Verification items for the finished model (mm, model axes). Coordinates: 2 decimals unless noted, no trailing zeros. Write each loop counter-clockwise with the first axis right and the second up, starting at its lowest first coordinate (ties: lowest second). Pieces come first, ordered by that corner, then holes. Notation, with made-up numbers: M 31.25,5 L 45.25,5 A26 cw 45.25,44 Z; hole C 71,20 d2. An arc over 180 degrees is marked long. One line per item, written item: value.
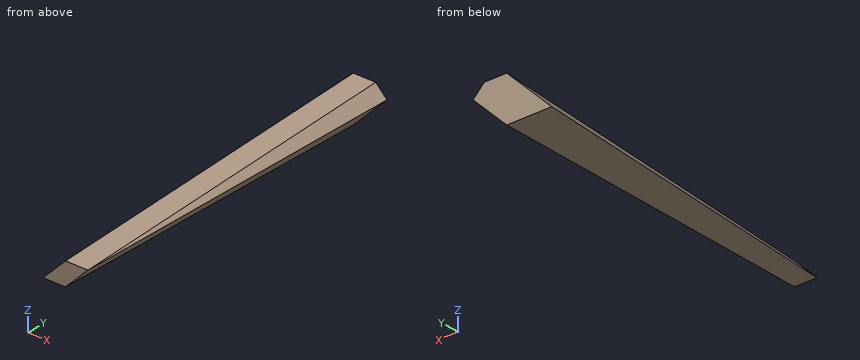
```python
from build123d import *

# Parameters (mm, degrees)
F0_W        = 10.16
F0_H        = 5.08
F1_DEPTH    = 38.1
F2_SIZE2    = 2.53999
F2_SIZE     = 38.09999
F3_T1_DEPTH = 64.3128613158
F4_T1_DEPTH = 13.0641595789
F4_T3_DEPTH = 44.702137425
F5_T1_DEPTH = 64.1438766671


# Not quite as in the source:
# - a fillet or chamfer that OpenCascade refuses, or shapes differently, is made with other operations: its cross-section is extruded or revolved along the edge and cut away or added
# - a fillet or chamfer is up to 0.001 mm smaller than in the source, because OpenCascade refuses the exact size


with BuildPart() as f1:
    # F0 (on Front) → F1 (new body)
    with BuildSketch(Plane.XZ):
        with Locations((5.08, 2.54)):
            Rectangle(F0_W, F0_H)
    extrude(amount=F1_DEPTH)

    # F2 (size 38.1 and 2.54 in the source; OpenCascade refuses exactly that, so slightly less here)
    f2_edges = [f1.edges().sort_by_distance(p)[0] for p in [
        (5.08, -38.1, 5.08),
    ]]
    f2_side = f1.faces().sort_by_distance((5.08, -19.05, 5.08))[0]
    chamfer(f2_edges, length=F2_SIZE, length2=F2_SIZE2, reference=f2_side)

    # F3: chamfer of 5.08 on 1 edges, made by hand

    # F3_s2 → F3_t1 (cut)
    with BuildSketch(Plane(origin=(0, 13.3723717196, 0.8914881722), x_dir=(1, 0, 0), z_dir=(0, -0.9977851741, -0.0665187672))):
        Polygon((0, -0.0112506505), (5.08, 5.0687493495), (0, 5.0687493495), align=None)
    extrude(amount=F3_T1_DEPTH, mode=Mode.SUBTRACT)

    # F4: chamfer of 2.54 on 2 edges, made by hand

    # F4_s2 → F4_t1 (cut)
    with BuildSketch(Plane.XZ.offset(-6.5320747894)):
        Polygon((7.62, 5.08), (10.16, 2.54), (10.16, 5.08), align=None)
    extrude(amount=F4_T1_DEPTH, mode=Mode.SUBTRACT)

    # F4_s4 → F4_t3 (cut)
    with BuildSketch(Plane(origin=(0, 0.3226895493, 0.0215125576), x_dir=(1, 0, 0), z_dir=(0, -0.9977851741, -0.0665187672))):
        Polygon((7.62, 5.0687493495), (10.16, 2.5287493495), (10.16, 5.0687493495), align=None)
    extrude(amount=F4_T3_DEPTH, mode=Mode.SUBTRACT)

    # F5: chamfer of 5.08 on 1 edges, made by hand

    # F5_s2 → F5_t1 (cut)
    with BuildSketch(Plane.XZ.offset(-13.0641495789)):
        Polygon((10.16, 5.08), (5.08, 0), (10.16, 0), align=None)
    extrude(amount=F5_T1_DEPTH, mode=Mode.SUBTRACT)


solid = f1.part
```
Item 1: Go/stop test with flat-tipped pins: P1, Ø3, axis at y = -33.5, z = 1.5, coming from the +X side; P2, Ø1.5, axis at y = -25, z = 3, coming from the -X side. Record where each tip stops, or that it passes through.
The answers:
P1: stops at x = 7.8
P2: stops at x = 3.92
Item 2: Cross-section at C-C, the plane z = 1.2. Enter the section's corners in (x, y), and give its area (3 significant figures).
The answers:
outline: M 1.21,0 L 3.74,-38.1 L 6.28,-38.1 L 6.28,0 Z
area: 145 mm²
Item 3: Cross-section at B-B, the plane y = -30. Enter the section's corners in (x, z).
The answers:
outline: M 2.01,0 L 5.08,0 L 7.89,2.81 L 7.62,3.08 L 5.08,3.08 Z
Item 4: Cross-section at D-D, the plane x = 3. Enter the section's corners in (y, z).
The answers:
outline: M -38.1,0 L 0,0 L 0,3 L -38.1,0.46 Z
Item 5: Scan lines: line 1 (Z direction, x = 5.75, y = -33.5); line 2 (X direction, y = -18, z = 2.8); line 3 (Z direction, x = 4, y = -4.5). Record each from-to range of solid material in increasing order.
The answers:
line 1: z = 0.67 to 2.85
line 2: x = 4 to 7.88
line 3: z = 0 to 3.7
